from build123d import *

# Parameters (mm, degrees)
BOSS_EXTRUDE1_DEPTH = 18.25625
SKETCH4_W           = 88.9
SKETCH4_H           = 88.9
BOSS_EXTRUDE2_DEPTH = 18.25625
CUT_EXTRUDE1_DEPTH  = 1003.285006268
FILLET1_R           = 3.3782


with BuildPart() as part:
    # Sketch3 → Boss-Extrude1 (new body)
    with BuildSketch(Plane(origin=(0, 0, 0), x_dir=(1, 0, 0), z_dir=(0, 1, 0))):
        with BuildLine():
            Line((-501.65, -501.65), (-590.55, -590.55))
            Line((-590.55, -590.55), (-553.84414606, -590.55))
            ThreePointArc((-553.84414606, -590.55), (0, -809.625), (553.84414606, -590.55))
            Line((553.84414606, -590.55), (590.55, -590.55))
            Line((590.55, -590.55), (501.65, -501.65))
            Line((501.65, -501.65), (501.65, -569.352841501))
            ThreePointArc((501.65, -569.352841501), (0, -758.825), (-501.65, -569.352841501))
            Line((-501.65, -569.352841501), (-501.65, -501.65))
        make_face()
    extrude(amount=BOSS_EXTRUDE1_DEPTH)

    # Sketch4 → Boss-Extrude2 (add)
    with BuildSketch(Plane(origin=(0, 18.25625, 0), x_dir=(1, 0, 0), z_dir=(0, 1, 0))):
        with Locations((-546.1, -546.1)):
            Rectangle(SKETCH4_W, SKETCH4_H)
        with Locations((546.1, -546.1)):
            Rectangle(SKETCH4_W, SKETCH4_H)
    extrude(amount=-BOSS_EXTRUDE2_DEPTH)

    # Sketch5 → Cut-Extrude1 (cut, through all)
    with BuildSketch(Plane(origin=(0, 18.25625, 0), x_dir=(1, 0, 0), z_dir=(0, 1, 0))):
        Polygon((-590.55, -590.55), (-501.65, -501.65), (-590.55, -501.65), align=None)
        Polygon((501.65, -501.65), (590.55, -590.55), (590.55, -501.65), align=None)
    extrude(amount=-CUT_EXTRUDE1_DEPTH, mode=Mode.SUBTRACT)

    # Fillet1
    fillet1_edges = [part.edges().sort_by_distance(p)[0] for p in [
        (-501.65, 9.128125, 569.352841501),
        (501.65, 9.128125, 569.352841501),
        (553.84414606, 9.128125, 590.55),
        (-553.84414606, 9.128125, 590.55),
    ]]
    fillet(fillet1_edges, radius=FILLET1_R)


solid = part.part
Geometry: final body of the model. Coordinates: model frame, mm. Give positions to 0.01 mm unless a question says otherwise; leave off trailing zeros. Order: outer loops, then holes, each group sorted by start corner. A loop starts at its lowest first (then second) coordinate and runs counter-clockwise, first axis right, second up. Notation, with made-up numbers: (1, 6.25) -> (40, 6.25) arc R11 ccw to (40, 27.25) -> close; hole circle Ø10 at (-8, 22.25). An arc over 180 degrees is marked (long way). Answer as a JSON object with one key per item and string values.
Q1. Section D-D (x = 79). Output: boundary loops of the cut face in (y, z), plus the area to 3 significant figures.
Entries:
{"outline": "(0, 754.7) -> (18.26, 754.7) -> (18.26, 805.76) -> (0, 805.76) -> close", "area": "932 mm^2"}
Q2. Section A-A (z = 539). Output: boundary loops of the cut face in (x, y).
Entries:
{"outline": "(-539, 0) -> (-501.65, 0) -> (-501.65, 18.26) -> (-539, 18.26) -> close; (501.65, 0) -> (539, 0) -> (539, 18.26) -> (501.65, 18.26) -> close"}
Q3. Section C-C (z = 652). Output: boundary loops of the cut face in (x, y), plus the area to 3 significant figures.
Entries:
{"outline": "(-479.99, 0) -> (-388.22, 0) -> (-388.22, 18.26) -> (-479.99, 18.26) -> close; (388.22, 0) -> (479.99, 0) -> (479.99, 18.26) -> (388.22, 18.26) -> close", "area": "3,350 mm^2"}
Q4. First-contact query: pin 1 (5 mm diameter, centred on x = -432.5, y = 7, fed in from +Z); pin 2 (5.5 mm diameter, centred on x = 577, y = 7.5, fed in from +Z); pin 3 (8 mm diameter, centred on x = 466.5, y = 3.5, fed in from +Z). Flat tips, straight axial feed; report the tip coordinate or a pass-through.
Entries:
{"pin 1": "stops at z = 686", "pin 2": "stops at z = 590.55", "pin 3": "stops at z = 664.52"}
Q5. Material intervals for probe 1 along X at (y, z) = (11.5, 584.5); probe 2 along X at (y, z) = (17.25, 653.5); probe 3 along Z at (x, y) = (368, 4), sorted ascending.
Entries:
{"probe 1": "x = -584.5 to -483.92, 483.92 to 584.5", "probe 2": "x = -477.94 to -385.69, 385.69 to 477.94", "probe 3": "z = 663.62 to 721.16"}
Q6. Draft query along X for faces 1 (the flat face through (-547, 9, 547)), 2 (the flat face through (-3, 18.256, 769)), 3 (the cylindrical face through (7.651, 9, 758.786)). Return one class per face: released by +X, released by -X, zero draft, split by the parting line, or undercut.
Entries:
{"face 1": "released by -X", "face 2": "zero draft", "face 3": "undercut"}
Q7. Section B-B (y = 4.5). Output: boundary loops of the cut face in (x, z) (3 decimals), plus the area to 3 significant figures.
Entries:
{"outline": "(-590.55, 590.55) -> (-501.65, 501.65) -> (-501.65, 567.825) arc R3.378 cw to (-500.5, 570.364) arc R758.825 cw to (500.5, 570.364) arc R3.378 cw to (501.65, 567.825) -> (501.65, 501.65) -> (590.55, 590.55) -> (555.179, 590.55) arc R3.378 cw to (552.872, 591.46) arc R809.625 ccw to (-552.872, 591.46) arc R3.378 cw to (-555.179, 590.55) -> close", "area": "65,600 mm^2"}
